from build123d import *

# Parameters (mm, degrees)
F0_W      = 63.5
F0_H      = 38.1
F1_DEPTH  = 7.62
F2_DEPTH  = 17.78
F3_W      = 6.35
F3_H      = 38.1
F3_W_2    = 5.6318170339
F4_DEPTH  = 17.78
F5_W      = 16.51
F5_H      = 20.32
F6_DEPTH  = 27.92324
F7_W      = 16.51
F7_H      = 20.32
F8_DEPTH  = 28.68757
F9_R      = 12.7
F10_DEPTH = 30.26185


with BuildPart() as f1:
    # F0 (on Front) → F1 (new body)
    with BuildSketch(Plane.XZ):
        with Locations((-0.6209928542, -0.4360526333)):
            Rectangle(F0_W, F0_H)
    extrude(amount=F1_DEPTH)

    # F2 (add): a face of the model
    f2_faces = [f1.faces().sort_by_distance(p)[0] for p in [
        (-0.6209928542, 0, -0.4360526333),
    ]]
    extrude(f2_faces, amount=F2_DEPTH)

    # F3 (on Front) → F4 (cut)
    with BuildSketch(Plane.XZ):
        with Locations((27.9540071458, -0.4360526333)):
            Rectangle(F3_W, F3_H)
        with Locations((-29.5550843373, -0.4360526333)):
            Rectangle(F3_W_2, F3_H)
    extrude(amount=-F4_DEPTH, mode=Mode.SUBTRACT)

    # F5 (on Front) → F6 (cut)
    with BuildSketch(Plane.XZ):
        with Locations((-24.1159928542, -9.3260526333)):
            Rectangle(F5_W, F5_H)
    extrude(amount=-F6_DEPTH, mode=Mode.SUBTRACT)

    # F7 (on Front) → F8 (cut)
    with BuildSketch(Plane.XZ):
        with Locations((22.8740071458, -9.3260526333)):
            Rectangle(F7_W, F7_H)
    extrude(amount=-F8_DEPTH, mode=Mode.SUBTRACT)

    # F9 (on face) → F10 (cut)
    with BuildSketch(Plane.XZ.offset(7.62)):
        with Locations((-0.6209928542, -19.4860526333)):
            Circle(F9_R)
    extrude(amount=-F10_DEPTH, mode=Mode.SUBTRACT)


solid = f1.part
Input: part model. Units: mm. Frame: model coordinates. A direction names the side the tool comes from. Coordinates: 2 decimals unless noted, no trailing zeros. Order: outer loops, then holes, each group sorted by start corner. A loop starts at its lowest first (then second) coordinate and runs counter-clockwise, first axis right, second up.
1. Access query for faces 1 (the flat face through (-15.861, 9, -9)), 2 (the flat face through (24.779, 9, 10)), 3 (the flat face through (-1, 5, 18.614)), 4 (the flat face through (-26.739, 9, 10)), 5 (the flat face through (25, 0, -4)). Directions: +Z, -Z, +X, -X, +Y, -Y. A direction counts if a zero-diameter tool reaches every point of the face in a straight line with its end or side. Return the directions, or none.
Checked values:
face 1: -Z, -X, +Y
face 2: +Z, -Z, +X, +Y
face 3: +Z, +X, -X, +Y, -Y
face 4: +Z, -Z, -X, +Y
face 5: -Z, +X, +Y
2. Cut plane B-B, the plane y = 14. Return loops of the section in (x, z), plus the area to 3 significant figures.
Checked values:
outline: (-26.74, 0.83) - (-15.86, 0.83) - (-15.86, -19.49) - (-13.32, -19.49) arc R12.7 cw to (12.08, -19.49) - (14.62, -19.49) - (14.62, 0.83) - (24.78, 0.83) - (24.78, 18.61) - (-26.74, 18.61) - close
area: 1,280 mm2
3. Cut plane A-A, the plane z = -14. Return loops of the section in (x, y).
Checked values:
outline: (-32.37, -7.62) - (-12.07, -7.62) - (-12.07, 17.78) - (-15.86, 17.78) - (-15.86, 0) - (-32.37, 0) - close; (10.83, -7.62) - (31.13, -7.62) - (31.13, 0) - (14.62, 0) - (14.62, 17.78) - (10.83, 17.78) - close
4. Cut plane D-D, the plane x = -18. Return loops of the section in (y, z), plus the area to 3 significant figures.
Checked values:
outline: (-7.62, -19.49) - (0, -19.49) - (0, 0.83) - (17.78, 0.83) - (17.78, 18.61) - (-7.62, 18.61) - close
area: 606 mm2
5. Cut plane C-C, the plane z = 12.5. Return loops of the section in (x, y).
Checked values:
outline: (-32.37, -7.62) - (31.13, -7.62) - (31.13, 0) - (24.78, 0) - (24.78, 17.78) - (-26.74, 17.78) - (-26.74, 0) - (-32.37, 0) - close
6. Contact query for flat-ended pins moving along their axis: P1, Ø5.5, axis at y = 8.5, z = -10, coming from the -X side; P2, Ø2, axis at x = 0.5, y = 13, coming from the -Z side; P3, Ø5.5, axis at y = 5, z = 13, coming from the -X side. Output: stop coordinate, or through.
Checked values:
P1: stops at x = -15.86
P2: stops at z = -6.96
P3: stops at x = -26.74
7. Ray query, line 1 along Z through (x, y) = (-19.5, 4.25); line 2 along Y through (x, z) = (-18, -4); line 3 along X through (y, z) = (15, 4). Return the intervals inside material, ascending.
Checked values:
line 1: z = 0.83 to 18.61
line 2: y = -7.62 to 0
line 3: x = -26.74 to 24.78
